Here's how the part is built. I have some questions about the finished solid (model axes, mm). A direction names the side the tool comes from. Coordinates: 2 decimals unless noted, no trailing zeros. Write each loop counter-clockwise with the first axis right and the second up, starting at its lowest first coordinate (ties: lowest second). Pieces come first, ordered by that corner, then holes. Notation, with made-up numbers: (50, 49.25) -> (73, 49.25) arc R5 cw to (73, 54.25) -> close; hole circle Ø5 at (73.5, 34.25). An arc over 180 degrees is marked (long way). Use CSV: the item, a comma, the result in double quotes. Start each with the question number.
```python
from build123d import *

# Parameters (mm, degrees)
SKETCH1_R           = 3
BOSS_EXTRUDE1_DEPTH = 20
SKETCH2_R           = 0.75
BOSS_EXTRUDE2_DEPTH = 10


with BuildPart() as part:
    # Sketch1 → Boss-Extrude1 (new body)
    with BuildSketch(Plane(origin=(0, 0, 0), x_dir=(1, 0, 0), z_dir=(0, 1, 0))):
        Circle(SKETCH1_R)
    extrude(amount=BOSS_EXTRUDE1_DEPTH)

    # Sketch2 → Boss-Extrude2 (add)
    with BuildSketch(Plane(origin=(0, 20, 0), x_dir=(1, 0, 0), z_dir=(0, 1, 0))):
        with Locations((1.5, 0)):
            Circle(SKETCH2_R)
        with Locations((-1.5, 0)):
            Circle(SKETCH2_R)
    extrude(amount=BOSS_EXTRUDE2_DEPTH)


solid = part.part
```
Item 1: I want a section at A-A on z = 0. Please give me the cut outline in (x, y).
Item 2: Thinking about a two-plate mould opening in X: for faces 1 (the cylindrical face through (-3, 10, 0)), 2 (the cylindrical face through (-0.785, 24.93, -0.225)), 3 (the flat face through (0, 0, 0)), 4 (the cylindrical face through (2.19, 24.93, 0.29)), which applies, +X half, -X half, draft (parallel to the pull), parting line (faces both ways), or undercut?
Item 3: If I drill on line 1 along X through (y, z) = (25.25, -0.1); line 2 along X through (y, z) = (2, -0.15); line 3 along Y through (x, z) = (1.7, -0.95), over which ranges is the centre line in solid material (lowest first)?
Item 4: I'm going to push flat-ended pins straight in: pin 1 (3 mm diameter, centred on y = 26, z = -0.5, fed in from -X); pin 2 (1 mm diameter, centred on y = 6.5, z = 1.5, fed in from -X). Where does each tip first touch, or does it pass through?
Item 5: I want a section at D-D on y = 5.25. Please give me the cut outline in (x, z), then the cut area to 3 significant figures.
Item 6: I want a section at C-C on x = 1.5. Please give me the cut outline in (y, z).
Item 7: I want a section at B-B on y = 26.5. Please give me the cut outline in (x, z).
Item 8: Which directions (+Z, -Z, +X, -X, +Y, -Y) give clear straight access to the entire face, cutting with the end or side of a thin tool? Please do faces 5 (the flat face through (1, 30, 0)), 6 (the flat face through (0, 20, 0)).
Geometry says:
1,outline,"(-3, 0) -> (3, 0) -> (3, 20) -> (2.25, 20) -> (2.25, 30) -> (0.75, 30) -> (0.75, 20) -> (-0.75, 20) -> (-0.75, 30) -> (-2.25, 30) -> (-2.25, 20) -> (-3, 20) -> close"
2,face 1,"parting line"
2,face 2,"undercut"
2,face 3,"draft"
2,face 4,"undercut"
3,line 1,"-2.24 to -0.76, 0.76 to 2.24"
3,line 2,"-3 to 3"
3,line 3,"0 to 20"
4,pin 1,"x = -2.25"
4,pin 2,"x = -2.83"
5,outline,"circle Ø6 at (0, 0)"
5,area,"28.3 mm2"
6,outline,"(0, -2.6) -> (20, -2.6) -> (20, -0.75) -> (30, -0.75) -> (30, 0.75) -> (20, 0.75) -> (20, 2.6) -> (0, 2.6) -> close"
7,outline,"circle Ø1.5 at (-1.5, 0); circle Ø1.5 at (1.5, 0)"
8,face 5,"+Z, -Z, +X, -X, +Y"
8,face 6,"+Y"
